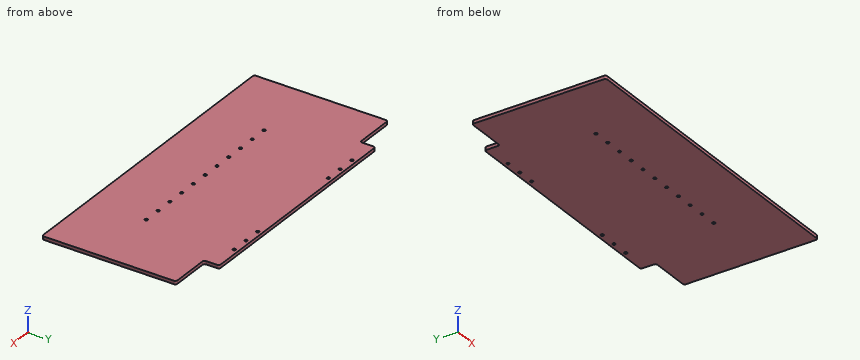
Autodesk Inventor part; units mm, degrees
ref_plane "YZ Plane" through (0, 0, 0) normal (1, 0, 0) x (0, 1, 0)
ref_plane "XZ Plane" through (0, 0, 0) normal (0, 1, 0) x (-1, 0, 0)
ref_plane "XY Plane" through (0, 0, 0) normal (0, 0, 1) x (1, 0, 0)
sketch "Sketch1" plane through (0, 0, 0) normal (0, 0, 1) x (1, 0, 0)
  line L0 (-228.6, -107.95) -> (228.6, -107.95)
  line L1 (168.402, 107.95) -> (-168.402, 107.95)
  line L2 (-171.577, 91.059) -> (-171.577, 109.9058)
  line L3 (-171.577, 91.059) -> (-173.736, 88.9)
  line L4 (-232.664, 88.9) -> (-173.736, 88.9)
  line L5 (-232.664, 88.9) -> (-234.823, 91.059)
  line L6 (-234.823, 109.9058) -> (-234.823, 91.059)
  line L7 (-171.577, 109.9058) -> (-234.823, 109.9058)
  circle A0 centre (-177.8, 101.6) radius 2.0701
  circle A1 centre (-190.5, 101.6) radius 2.0701
  circle A2 centre (-203.2, 101.6) radius 2.0701
  circle A3 centre (-215.9, 101.6) radius 2.0701
  circle A4 centre (-228.6, 101.6) radius 2.0701
  line L8 (234.823, 109.9058) -> (234.823, 91.059)
  line L9 (234.823, 91.059) -> (232.664, 88.9)
  line L10 (173.736, 88.9) -> (232.664, 88.9)
  line L11 (173.736, 88.9) -> (171.577, 91.059)
  line L12 (171.577, 109.9058) -> (171.577, 91.059)
  line L13 (234.823, 109.9058) -> (171.577, 109.9058)
  circle A5 centre (177.8, 101.6) radius 2.0701
  circle A6 centre (190.5, 101.6) radius 2.0701
  circle A7 centre (203.2, 101.6) radius 2.0701
  circle A8 centre (215.9, 101.6) radius 2.0701
  circle A9 centre (228.6, 101.6) radius 2.0701
  line L14 (168.402, 107.95) -> (168.402, 85.725)
  line L15 (168.402, 85.725) -> (228.6, 85.725)
  line L16 (-168.402, 107.95) -> (-168.402, 85.725)
  line L17 (-168.402, 85.725) -> (-228.6, 85.725)
  line L18 (-228.6, 85.725) -> (-228.6, -107.95)
  line L19 (228.6, -107.95) -> (228.6, 85.725)
  point P0 (0, 0)
  dimension "d4" = 3.175
  dimension "d5" = 3.175
  dimension "d6" = 3.175
  dimension "d7" = 3.175
  dimension "d8" = 457.2
  dimension "d9" = 215.9
extrude "Extrusion1" add sketch "Sketch1" along normal blind 4.7625 contours L18 L17 L16 L1 L14 L15 L19 L0
fillet "Fillet1" radius 3.175 8 edges at (228.6, -107.95, 2.3813) (168.402, 107.95, 2.3813) (168.402, 85.725, 2.3813) (228.6, 85.725, 2.3813) (-168.402, 107.95, 2.3813) (-168.402, 85.725, 2.3813) (-228.6, 85.725, 2.3813) (-228.6, -107.95, 2.3813)
sketch "Sketch2" plane through (0, 0, 0) normal (0, 0, -1) x (-1, 0, 0)
  arc A0 (103.6687, -25.2476) -> (99.5313, -25.2476) centre (101.6, -25.3238) ccw
  line L0 (78.2687, -25.2476) -> (99.5313, -25.2476)
  arc A1 (78.2687, -25.2476) -> (74.1313, -25.2476) centre (76.2, -25.3238) ccw
  line L1 (52.8687, -25.2476) -> (74.1313, -25.2476)
  arc A2 (52.8687, -25.2476) -> (48.7313, -25.2476) centre (50.8, -25.3238) ccw
  line L2 (27.4687, -25.2476) -> (48.7313, -25.2476)
  arc A3 (27.4687, -25.2476) -> (23.3313, -25.2476) centre (25.4, -25.3238) ccw
  line L3 (2.0687, -25.2476) -> (23.3313, -25.2476)
  arc A4 (2.0687, -25.2476) -> (-2.0687, -25.2476) centre (0, -25.3238) ccw
  line L4 (-23.3313, -25.2476) -> (-2.0687, -25.2476)
  arc A5 (-23.3313, -25.2476) -> (-27.4687, -25.2476) centre (-25.4, -25.3238) ccw
  line L5 (-48.7313, -25.2476) -> (-27.4687, -25.2476)
  arc A6 (-48.7313, -25.2476) -> (-52.8687, -25.2476) centre (-50.8, -25.3238) ccw
  line L6 (-74.1313, -25.2476) -> (-52.8687, -25.2476)
  arc A7 (-74.1313, -25.2476) -> (-78.2687, -25.2476) centre (-76.2, -25.3238) ccw
  line L7 (-99.5313, -25.2476) -> (-78.2687, -25.2476)
  arc A8 (-99.5313, -25.2476) -> (-103.6687, -25.2476) centre (-101.6, -25.3238) ccw
  line L8 (-124.9313, -25.2476) -> (-103.6687, -25.2476)
  arc A9 (-124.9313, -25.2476) -> (-129.0687, -25.2476) centre (-127, -25.3238) ccw
  line L9 (-355.6, -25.2476) -> (-129.0687, -25.2476)
  line L10 (-355.6, -12.6238) -> (-355.6, -25.2476)
  line L11 (355.6, -12.6238) -> (-355.6, -12.6238)
  line L12 (355.6, -25.2476) -> (355.6, -12.6238)
  line L13 (129.0687, -25.2476) -> (355.6, -25.2476)
  arc A10 (129.0687, -25.2476) -> (124.9313, -25.2476) centre (127, -25.3238) ccw
  line L14 (103.6687, -25.2476) -> (124.9313, -25.2476)
  arc A11 (-99.5313, 101.7524) -> (-103.6687, 101.7524) centre (-101.6, 101.6762) ccw
  line L15 (-124.9313, 101.7524) -> (-103.6687, 101.7524)
  arc A12 (-124.9313, 101.7524) -> (-129.0687, 101.7524) centre (-127, 101.6762) ccw
  line L16 (-175.7355, 101.7524) -> (-129.0687, 101.7524)
  arc A13 (-175.7355, 101.7524) -> (-179.8645, 101.7524) centre (-177.8, 101.6) ccw
  line L17 (-188.4355, 101.7524) -> (-179.8645, 101.7524)
  arc A14 (-188.4355, 101.7524) -> (-192.5645, 101.7524) centre (-190.5, 101.6) ccw
  line L18 (-201.1355, 101.7524) -> (-192.5645, 101.7524)
  arc A15 (-201.1355, 101.7524) -> (-205.2645, 101.7524) centre (-203.2, 101.6) ccw
  line L19 (-213.8355, 101.7524) -> (-205.2645, 101.7524)
  arc A16 (-213.8355, 101.7524) -> (-217.9645, 101.7524) centre (-215.9, 101.6) ccw
  line L20 (-226.5355, 101.7524) -> (-217.9645, 101.7524)
  arc A17 (-226.5355, 101.7524) -> (-230.6645, 101.7524) centre (-228.6, 101.6) ccw
  line L21 (-355.6, 101.7524) -> (-230.6645, 101.7524)
  line L22 (-355.6, 114.3) -> (-355.6, 101.7524)
  line L23 (355.6, 114.3) -> (-355.6, 114.3)
  line L24 (355.6, 101.7524) -> (355.6, 114.3)
  line L25 (230.6645, 101.7524) -> (355.6, 101.7524)
  arc A18 (230.6645, 101.7524) -> (226.5355, 101.7524) centre (228.6, 101.6) ccw
  line L26 (217.9645, 101.7524) -> (226.5355, 101.7524)
  arc A19 (217.9645, 101.7524) -> (213.8355, 101.7524) centre (215.9, 101.6) ccw
  line L27 (205.2645, 101.7524) -> (213.8355, 101.7524)
  arc A20 (205.2645, 101.7524) -> (201.1355, 101.7524) centre (203.2, 101.6) ccw
  line L28 (192.5645, 101.7524) -> (201.1355, 101.7524)
  arc A21 (192.5645, 101.7524) -> (188.4355, 101.7524) centre (190.5, 101.6) ccw
  line L29 (179.8645, 101.7524) -> (188.4355, 101.7524)
  arc A22 (179.8645, 101.7524) -> (175.7355, 101.7524) centre (177.8, 101.6) ccw
  line L30 (129.0687, 101.7524) -> (175.7355, 101.7524)
  arc A23 (129.0687, 101.7524) -> (124.9313, 101.7524) centre (127, 101.6762) ccw
  line L31 (103.6687, 101.7524) -> (124.9313, 101.7524)
  arc A24 (103.6687, 101.7524) -> (99.5313, 101.7524) centre (101.6, 101.6762) ccw
  line L32 (78.2687, 101.7524) -> (99.5313, 101.7524)
  arc A25 (78.2687, 101.7524) -> (74.1313, 101.7524) centre (76.2, 101.6762) ccw
  line L33 (64.0989, 101.7524) -> (74.1313, 101.7524)
  spline S0 degree 2 poles (64.0989, 101.7524) (63.534, 102.6488) (62.8722, 103.4567) knots 1.72164 1.72164 1.72164 2 2 2
  spline S1 degree 2 poles (62.8722, 103.4567) (60.4022, 106.3898) (53.1156, 109.5391) (47.8051, 109.5391) knots 0 0 0 1 2 2 2
  spline S2 degree 2 poles (47.8051, 109.5391) (46.0143, 109.5391) (42.1241, 109.076) (41.4757, 108.8907) knots 0 0 0 1 2 2 2
  line L34 (41.4757, 108.8907) -> (41.4757, 101.7524)
  line L35 (33.0922, 101.7524) -> (41.4757, 101.7524)
  spline S3 degree 2 poles (33.0922, 101.7524) (32.0797, 104.0718) (30.2062, 105.7723) knots 1.066482 1.066482 1.066482 2 2 2
  spline S4 degree 2 poles (30.2062, 105.7723) (28.1994, 107.5939) (22.7036, 109.6008) (18.6898, 109.6008) knots 0 0 0 1 2 2 2
  spline S5 degree 2 poles (18.6898, 109.6008) (14.429, 109.57) (8.3157, 108.1806) (6.3088, 107.2852) knots 0 0 0 1 2 2 2
  line L36 (6.3088, 107.2852) -> (6.3088, 101.7524)
  line L37 (-0.2839, 101.7524) -> (6.3088, 101.7524)
  spline S6 degree 2 poles (-0.2839, 101.7524) (-1.2964, 104.0718) (-3.1699, 105.7723) knots 1.066482 1.066482 1.066482 2 2 2
  spline S7 degree 2 poles (-3.1699, 105.7723) (-5.1767, 107.5939) (-10.6725, 109.6008) (-14.6863, 109.6008) knots 0 0 0 1 2 2 2
  spline S8 degree 2 poles (-14.6863, 109.6008) (-18.9471, 109.57) (-25.0604, 108.1806) (-27.0673, 107.2852) knots 0 0 0 1 2 2 2
  line L38 (-27.0673, 107.2852) -> (-27.0673, 101.7524)
  line L39 (-41.1772, 101.7524) -> (-27.0673, 101.7524)
  line L40 (-41.1772, 101.7524) -> (-41.1772, 102.1599)
  line L41 (-41.1772, 102.1599) -> (-33.3349, 102.1599)
  line L42 (-33.3349, 102.1599) -> (-33.3349, 108.7981)
  line L43 (-33.3349, 108.7981) -> (-58.4982, 108.7981)
  line L44 (-58.4982, 108.7981) -> (-58.4982, 102.1599)
  line L45 (-58.4982, 102.1599) -> (-50.4707, 102.1599)
  line L46 (-50.4707, 102.1599) -> (-50.4707, 101.7524)
  line L47 (-74.1313, 101.7524) -> (-50.4707, 101.7524)
  arc A26 (-74.1313, 101.7524) -> (-78.2687, 101.7524) centre (-76.2, 101.6762) ccw
  line L48 (-99.5313, 101.7524) -> (-78.2687, 101.7524)
  point P0 (0, 0)
hole "Hole1" at (-127, 101.6762, 0) at (-101.6, 101.6762, 0) at (-76.2, 101.6762, 0) at (76.2, 101.6762, 0) at (101.6, 101.6762, 0) at (127, 101.6762, 0) at (-127, -25.3238, 0) at (-101.6, -25.3238, 0) at (-76.2, -25.3238, 0) at (-50.8, -25.3238, 0) at (-25.4, -25.3238, 0) at (0, -25.3238, 0) at (25.4, -25.3238, 0) at (50.8, -25.3238, 0) at (76.2, -25.3238, 0) at (101.6, -25.3238, 0) at (127, -25.3238, 0) direction (0, 0, 1) diameter 4.1402 end through all
sketch "Sketch4" plane through (0, 0, 0) normal (0, 0, -1) x (-1, 0, 0)
  line L0 (-165.227, 107.95) -> (165.227, 107.95)
  line L1 (107.95, -107.95) -> (-107.95, -107.95) construction
  line L2 (-107.95, -107.95) -> (-107.95, 107.95) construction
  line L3 (-107.95, 107.95) -> (107.95, 107.95) construction
  line L4 (107.95, 107.95) -> (107.95, -107.95) construction
  line L5 (197.0019, -39.6304) -> (129.4704, -39.6304) construction
  line L6 (129.4704, -39.6304) -> (129.4704, 38.94) construction
  line L7 (129.4704, 38.94) -> (197.0019, 38.94) construction
  line L8 (197.0019, 38.94) -> (197.0019, -39.6304) construction
  line L9 (-125.3858, -27.2271) -> (-180.4191, -27.2271) construction
  line L10 (-180.4191, -27.2271) -> (-180.4191, 36.8021) construction
  line L11 (-180.4191, 36.8021) -> (-125.3858, 36.8021) construction
  line L12 (-125.3858, 36.8021) -> (-125.3858, -27.2271) construction
  line L13 (-51.4537, 12.8385) -> (-125.3858, 12.8385) construction
  line L14 (-125.3858, 12.8385) -> (-125.3858, -68.9649) construction
  line L15 (-125.3858, -68.9649) -> (-51.4537, -68.9649) construction
  line L16 (-51.4537, -68.9649) -> (-51.4537, 12.8385) construction
  line L17 (225.425, -107.95) -> (-225.425, -107.95)
  line L18 (-228.6, -104.775) -> (-228.6, 82.55)
  point P0 (0, 0)
decal "Decal1"
decal "Decal2"
decal "Decal3"
properties part number "C17_TK_VerticalElectricBoard" material "Polycarbonate, Clear"
For this review, take the finished solid that the model builds, in its own axes (mm). Give positions to 0.01 mm unless a question says otherwise; leave off trailing zeros.
Item 1: For line 1 along Y through (x, z) = (-101.6, 2.4); line 2 along Y through (x, z) = (25.4, 2.9); line 3 along Y through (x, z) = (75.5, 0.65), list the stretches that pass through material, from the lowest coordinate up.
Item 2: Take a section at A-A, the plane z = 1.65. Give the number of separate pieces and of enclosed holes in the cut face, and give its area (3 significant figures).
Item 3: Insertion check: pin 1 (2.5 mm diameter, centred on x = -101.6, y = 101.68, fed in from +Z); pin 2 (2.5 mm diameter, centred on y = 94, z = 1.5, fed in from -X); pin 3 (1.4 mm diameter, centred on x = 196, z = 2.5, fed in from +Y) (3 decimals). Each pin has a flat end and moves straight along its axis. Give the tip position at first contact, or say it passes through.
Calculated:
1. line 1: y = -107.95 to -27.39, -23.25 to 99.61, 103.75 to 107.95
1. line 2: y = -107.95 to -27.39, -23.25 to 107.95
1. line 3: y = -107.95 to -27.27, -23.38 to 99.73, 103.62 to 107.95
2. separate pieces: 1
2. enclosed holes: 17
2. area: 95,800 mm2
3. pin 1: passes through
3. pin 2: stops at x = -168.4
3. pin 3: stops at y = 85.725
